Part print with two shaded views. Sizes in mm from the minimum x, y, z corner. A direction names the side the tool comes from. Round coordinates to 2 decimals unless told otherwise and drop trailing zeros. Order: outer loops, then holes, each group sorted by start corner. A loop starts at its lowest first (then second) coordinate and runs counter-clockwise, first axis right, second up. Notation, with made-up numbers: (40.5, 85) - (54.5, 85) arc R27 ccw to (54.5, 102) - close; hole circle Ø5 at (-28.75, 74). An arc over 180 degrees is marked (long way). Answer as CSV lines item,"result". Start each with the question number.
1. Band-saw the part on D-D on z = 5.5. List the corners of the cut face in (x, y), then the cut area to 3 significant figures.
2. Pin check, flat tips, straight feed: pin 1 Ø6 at (y, z) = (68, 17.5) entering from +X; pin 2 Ø12 at (x, z) = (42, 14.5) entering from +Y. Stop position of each tip, or through.
3. Band-saw the part on A-A on x = 60. List the corners of the cut face in (y, z), then the cut area to 3 significant figures.
4. Band-saw the part on B-B on z = 18. List the corners of the cut face in (x, y), then the cut area to 3 significant figures.
5. Pull direction Z, two halves, no side cores. Call the marked faces 1, 2 and 3: released by +Z, released by -Z, zero draft, split by the parting line, or undercut.
6. 3-axis set-ups, long thin cutter, end or side, ignore diameter. For the marked faces 4 and 5: which of +Z, -Z, +X, -X, +Y, -Y reach the whole face in a straight line?
7. Wall check: line 1 along Z through (x, y) = (20, 2.75); line 2 along X through (y, z) = (2.25, 18); line 3 along X through (y, z) = (47.5, 20.5). Give the ranges that are in metal, low to high. Write a range as [from, to].
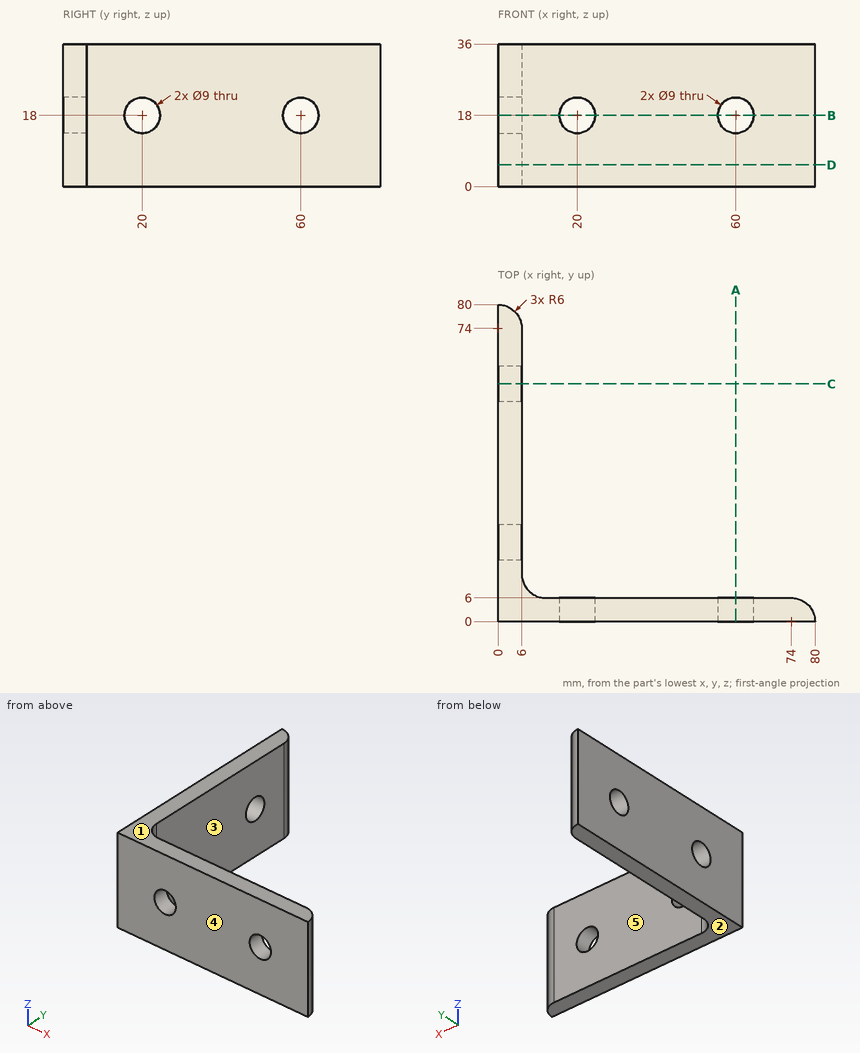
Reply:
1,outline,"(0, 0) - (80, 0) arc R6 ccw to (74, 6) - (12, 6) arc R6 cw to (6, 12) - (6, 74) arc R6 ccw to (0, 80) - close"
1,area,"916 mm2"
2,pin 1,"stops at x = 6"
2,pin 2,"stops at y = 6"
3,outline,"(0, 0) - (6, 0) - (6, 13.5) - (0, 13.5) - close; (0, 22.5) - (6, 22.5) - (6, 36) - (0, 36) - close"
3,area,"162 mm2"
4,outline,"(0, 0) - (15.5, 0) - (15.5, 6) - (12, 6) arc R6 cw to (6, 12) - (6, 15.5) - (0, 15.5) - close; (0, 24.5) - (6, 24.5) - (6, 55.5) - (0, 55.5) - close; (0, 64.5) - (6, 64.5) - (6, 74) arc R6 ccw to (0, 80) - close; (24.5, 0) - (55.5, 0) - (55.5, 6) - (24.5, 6) - close; (64.5, 0) - (80, 0) arc R6 ccw to (74, 6) - (64.5, 6) - close"
4,area,"700 mm2"
5,face 1,"released by +Z"
5,face 2,"released by -Z"
5,face 3,"zero draft"
6,face 4,"+Z, -Z, +X, -X, -Y"
6,face 5,"+Z, -Z, +X, +Y"
7,line 1,"z = [0, 13.5], [22.5, 36]"
7,line 2,"x = [0, 15.5], [24.5, 55.5], [64.5, 79.56]"
7,line 3,"x = [0, 6]"
